Can you work these out from the model? Positions are in its coordinate system, mm. Face numbers are marked on the shaded views. A direction names the side the tool comes from. Give positions to 0.01 mm unless a question says otherwise; leave off trailing zeros. Order: outer loops, then holes, each group sorted by start corner. A loop starts at its lowest first (then second) coordinate and runs counter-clockwise, first axis right, second up. Notation, with made-up numbers: M 44.25,24 L 101.25,24 A31 cw 101.25,52 Z; hole C -35,37 d2. An arc over 180 degrees is marked long. Answer as a JSON object with one key per item and string values.
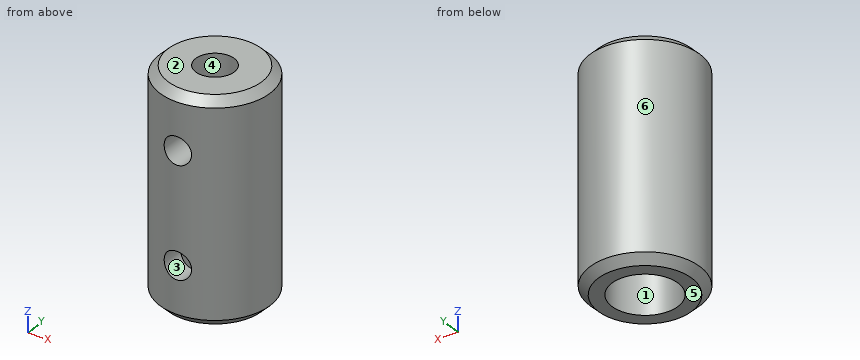
```python
from build123d import *

# Parameters (mm, degrees)
SKETCH1_R           = 10
SKETCH1_R_2         = 3.5
BOSS_EXTRUDE1_DEPTH = 40
CHAMFER1_SIZE       = 1.5
SKETCH2_R           = 6
CUT_EXTRUDE1_DEPTH  = 25
SKETCH3_R           = 2.5
CUT_EXTRUDE2_DEPTH  = 20


with BuildPart() as part:
    # Sketch1 → Boss-Extrude1 (new body)
    with BuildSketch(Plane.XY):
        Circle(SKETCH1_R)
        Circle(SKETCH1_R_2, mode=Mode.SUBTRACT)
    extrude(amount=BOSS_EXTRUDE1_DEPTH)

    # Chamfer1
    chamfer1_edges = [part.edges().sort_by_distance(p)[0] for p in [
        (-10, 0, 0),
        (-10, 0, 40),
    ]]
    chamfer(chamfer1_edges, length=CHAMFER1_SIZE)

    # Sketch2 → Cut-Extrude1 (cut)
    with BuildSketch(Plane(origin=(0, 0, 0), x_dir=(-1, 0, 0), z_dir=(0, 0, -1))):
        Circle(SKETCH2_R)
    extrude(amount=-CUT_EXTRUDE1_DEPTH, mode=Mode.SUBTRACT)

    # Sketch3 → Cut-Extrude2 (cut)
    with BuildSketch(Plane(origin=(0, 0, 0), x_dir=(1, 0, 0), z_dir=(0, 1, 0))):
        with Locations(Location((0, -10, 0), (0, 0, 270))):
            Circle(SKETCH3_R)
        with Locations(Location((0, -30, 0), (0, 0, 270))):
            Circle(SKETCH3_R)
    extrude(amount=-CUT_EXTRUDE2_DEPTH, mode=Mode.SUBTRACT)


solid = part.part
```
1) I want a section at D-D on z = 30. Write out the boundary of the cut face in (x, y), and give its area (3 significant figures).
Results found:
{"outline": "M -2.5,-9.68 L -2.5,-2.45 A3.5 cw long 2.5,-2.45 L 2.5,-9.68 A10 ccw long Z", "area": "242 mm²"}
2) I want a section at C-C on z = 37.5. Write out the boundary of the cut face in (x, y).
Results found:
{"outline": "C 0,0 d20; hole C 0,0 d7"}
3) Thinking about a two-plate mould opening in Y: for the marked faces 4, 5 and 6, which applies, pulls with the +Y half, pulls with the -Y half, needs draft (parallel to the pull), parting line crosses it, or undercut?
Results found:
{"face 4": "undercut", "face 5": "needs draft", "face 6": "parting line crosses it"}
4) I want a section at A-A on y = 0. Write out the boundary of the cut face in (x, z), and give its area (4 significant figures).
Results found:
{"outline": "M -10,1.5 L -8.5,0 L -6,0 L -6,25 L -3.5,25 L -3.5,40 L -8.5,40 L -10,38.5 Z; M 3.5,25 L 6,25 L 6,0 L 8.5,0 L 10,1.5 L 10,38.5 L 8.5,40 L 3.5,40 Z", "area": "390.5 mm²"}
5) I need wall thicknesses on L1, parallel to Y at x = 0, z = 14; L2, parallel to Y at x = 0, z = 34; L3, parallel to Z at x = 2, y = 4.5. Which ranges of each line are inside material? Lowest first, please.
Results found:
{"L1": "y = -10 to -6, 6 to 10", "L2": "y = -10 to -3.5, 3.5 to 10", "L3": "z = 25 to 40"}
6) I want a section at B-B on x = 0. Write out the boundary of the cut face in (y, z).
Results found:
{"outline": "M -10,1.5 L -8.5,0 L -6,0 L -6,7.5 L -10,7.5 Z; M -10,12.5 L -6,12.5 L -6,25 L -3.5,25 L -3.5,27.5 L -10,27.5 Z; M -10,32.5 L -3.5,32.5 L -3.5,40 L -8.5,40 L -10,38.5 Z; M 3.5,25 L 6,25 L 6,0 L 8.5,0 L 10,1.5 L 10,38.5 L 8.5,40 L 3.5,40 Z"}
7) I'm going to push flat-ended pins straight in: pin 1 Ø5 at (y, z) = (-6.5, 29) entering from -X; pin 2 Ø5 at (y, z) = (-5, 18) entering from +X; pin 3 Ø11 at (x, y) = (0, 0) entering from -Z; pin 4 Ø10 at (y, z) = (-3, 34.5) entering from +X. Where does each tip first touch, or does it pass through?
Results found:
{"pin 1": "stops at x = -9.17", "pin 2": "stops at x = 9.68", "pin 3": "stops at z = 25", "pin 4": "stops at x = 10"}
8) For the marked faces 1, 2 and 3, which set-ups out of +Z, -Z, +X, -X, +Y, -Y let a thin tool reach every point of the face, with its end or its side?
Results found:
{"face 1": "-Z", "face 2": "+Z, +X, -X, +Y, -Y", "face 3": "-Y"}
